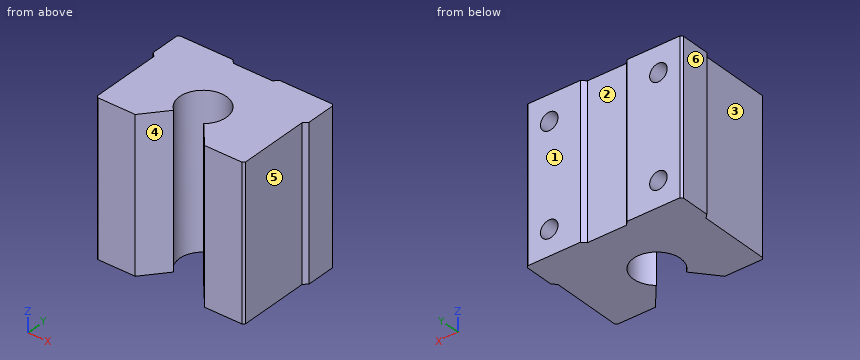
```python
from build123d import *

# Parameters (mm, degrees)
EXTRUDE1_DEPTH = 39
SKETCH2_R      = 2.25
EXTRUDE2_DEPTH = 10


with BuildPart() as part:
    # Sketch1 → Extrude1 (new body)
    with BuildSketch(Plane.XY):
        with BuildLine():
            Line((-18.5, -13.8), (-8.89445609, -13.8))
            Line((-8.89445609, -13.8), (-3.856725658, -7.796266659))
            ThreePointArc((-3.856725658, -7.796266659), (0, 2.8), (3.856725658, -7.796266659))
            Line((3.856725658, -7.796266659), (8.89445609, -13.8))
            Line((8.89445609, -13.8), (18.5, -13.8))
            Line((18.5, -13.8), (19, -13.3))
            Line((19, -13.3), (19, 4.8))
            Line((19, 4.8), (20, 5.8))
            Line((20, 5.8), (20, 13.3))
            Line((20, 13.3), (19.5, 13.8))
            Line((19.5, 13.8), (6, 13.8))
            Line((6, 13.8), (5, 12.8))
            Line((5, 12.8), (-5, 12.8))
            Line((-5, 12.8), (-6, 13.8))
            Line((-6, 13.8), (-19.5, 13.8))
            Line((-19.5, 13.8), (-20, 13.3))
            Line((-20, 13.3), (-20, 5.8))
            Line((-20, 5.8), (-19, 4.8))
            Line((-19, 4.8), (-19, -13.3))
            Line((-19, -13.3), (-18.5, -13.8))
        make_face()
    extrude(amount=EXTRUDE1_DEPTH)

    # Sketch2 → Extrude2 (cut)
    with BuildSketch(Plane(origin=(0, 13.8, 0), x_dir=(1, 0, 0), z_dir=(0, 1, 0))):
        with Locations((-14, -6.5)):
            Circle(SKETCH2_R)
        with Locations((-14, -32.5)):
            Circle(SKETCH2_R)
        with Locations((14, -32.5)):
            Circle(SKETCH2_R)
        with Locations((14, -6.5)):
            Circle(SKETCH2_R)
    extrude(amount=-EXTRUDE2_DEPTH, mode=Mode.SUBTRACT)


solid = part.part
```
Verification items for the finished model (mm, model axes). Face numbers are marked on the shaded views. A direction names the side the tool comes from. Give positions to 0.01 mm unless a question says otherwise; leave off trailing zeros. Loops run counter-clockwise (first coordinate to the right, second up) from the corner with the lowest first, then second, coordinate; pieces in that order, holes last.
1. Section check C-C, the plane z = 32.5. Enter the section's corners in (x, y).
2. Section check A-A, the plane y = -3.2. Enter the section's corners in (x, z), then the cut area to 3 significant figures.
3. Go/stop test with flat-tipped pins: pin 1 Ø12 at (y, z) = (-5, 22) entering from +X; pin 2 Ø6 at (x, z) = (-14, 32.5) entering from +Y; pin 3 Ø9 at (y, z) = (-8, 24) entering from -X; pin 4 Ø1.3 at (x, z) = (14.5, 7) entering from +Y. Record where each tip stops, or that it passes through.
4. Mould release check, pull along X, two halves, no side actions. Record for the marked faces 1, 2 and 3: released by +X, released by -X, zero draft, split by the parting line, or undercut.
5. Section check D-D, the plane y = 8.5. Enter the section's corners in (x, z), then the cut area to 3 significant figures.
6. Section check B-B, the plane x = 14. Enter the section's corners in (y, z), then the cut area to 3 significant figures.
7. Thickness scan on line 1 (X direction, y = 7.5, z = 32.5); line 2 (Z direction, x = -14, y = 10.5); line 3 (X direction, y = -3, z = 27). Record the ranges inside material, lowest first.
8. Set-up check for the marked faces 4, 5 and 6: record each of +Z, -Z, +X, -X, +Y, -Y from which the full face is reachable in a straight line by a thin tool's end or side.
Geometry says:
1. outline: (-20, 5.8) - (-19, 4.8) - (-19, -13.3) - (-18.5, -13.8) - (-8.89, -13.8) - (-3.86, -7.8) arc R6 cw (long way) to (3.86, -7.8) - (8.89, -13.8) - (18.5, -13.8) - (19, -13.3) - (19, 4.8) - (20, 5.8) - (20, 13.3) - (19.5, 13.8) - (16.25, 13.8) - (16.25, 3.8) - (11.75, 3.8) - (11.75, 13.8) - (6, 13.8) - (5, 12.8) - (-5, 12.8) - (-6, 13.8) - (-11.75, 13.8) - (-11.75, 3.8) - (-16.25, 3.8) - (-16.25, 13.8) - (-19.5, 13.8) - (-20, 13.3) - close
2. outline: (-19, 0) - (-6, 0) - (-6, 39) - (-19, 39) - close; (6, 0) - (19, 0) - (19, 39) - (6, 39) - close
2. area: 1,010 mm2
3. pin 1: stops at x = 19
3. pin 2: stops at y = 13.8
3. pin 3: stops at x = -19
3. pin 4: stops at y = 3.8
4. face 1: zero draft
4. face 2: undercut
4. face 3: released by -X
5. outline: (-20, 0) - (20, 0) - (20, 39) - (-20, 39) - close; hole circle Ø4.5 at (-14, 6.5); hole circle Ø4.5 at (-14, 32.5); hole circle Ø4.5 at (14, 6.5); hole circle Ø4.5 at (14, 32.5)
5. area: 1,500 mm2
6. outline: (-13.8, 0) - (13.8, 0) - (13.8, 4.25) - (3.8, 4.25) - (3.8, 8.75) - (13.8, 8.75) - (13.8, 30.25) - (3.8, 30.25) - (3.8, 34.75) - (13.8, 34.75) - (13.8, 39) - (-13.8, 39) - close
6. area: 986 mm2
7. line 1: x = -20 to -16.25, -11.75 to 11.75, 16.25 to 20
7. line 2: z = 0 to 4.25, 8.75 to 30.25, 34.75 to 39
7. line 3: x = -19 to -6, 6 to 19
8. face 4: +Z, -Z, -Y
8. face 5: +Z, -Z, +X, -Y
8. face 6: +Z, -Z, -X, +Y, -Y
